Design review of the part shown in the three views and the two pictorial views. Dimensions are in mm from the part's minimum x, y and z. A direction names the side the tool comes from. Round coordinates to 2 decimals unless told otherwise and drop trailing zeros. Write each loop counter-clockwise with the first axis right and the second up, starting at its lowest first coordinate (ties: lowest second). Pieces come first, ordered by that corner, then holes. Notation, with made-up numbers: (10.5, -4) -> (24.5, -4) arc R26 cw to (24.5, 13) -> close; hole circle Ø5 at (-39.75, 50). An arc over 180 degrees is marked (long way). Return JSON: item names as keys, results as strings. Group by question number.
1. Take a section at A-A, the plane y = 6. Give the number of separate pieces and of enclosed holes in the cut face, then the cut area to 3 significant figures.
2. Tool access review of the marked faces 1 and 2: name each direction out of +Z, -Z, +X, -X, +Y, -Y from which nothing blocks a thin tool from reaching the whole face with its end or side.
3. Take a section at C-C, the plane z = 8.75. Write out the cut boundary in (x, y), then the cut area to 3 significant figures.
4. Clearance check with flat-ended pins moving along their axes: P1, Ø3.5, axis at x = 19.5, z = 7, coming from the -Y side; P2, Ø2.5, axis at x = 7, z = 5.5, coming from the +Y side; P3, Ø1, axis at y = 2, z = 1.5, coming from the -X side. State where each tip first meets the part, or that it passes through.
5. Mouldability with a two-part tool opening along X and no side actions: class the marked faces 3, 4 and 5 as pulls with the +X half, pulls with the -X half, needs draft (parallel to the pull), parting line crosses it, or undercut.
6. For line 1 along X through (y, z) = (13, 7); line 2 along Z through (x, y) = (19.5, 12.3); line 3 along X through (y, z) = (3.75, 6.25) (1 decimal), list the stretches that pass through material, from the lowest coordinate up. Write a range as from..to.
7. Take a section at B-B, the plane x = 13. Write out the cut boundary in (y, z).
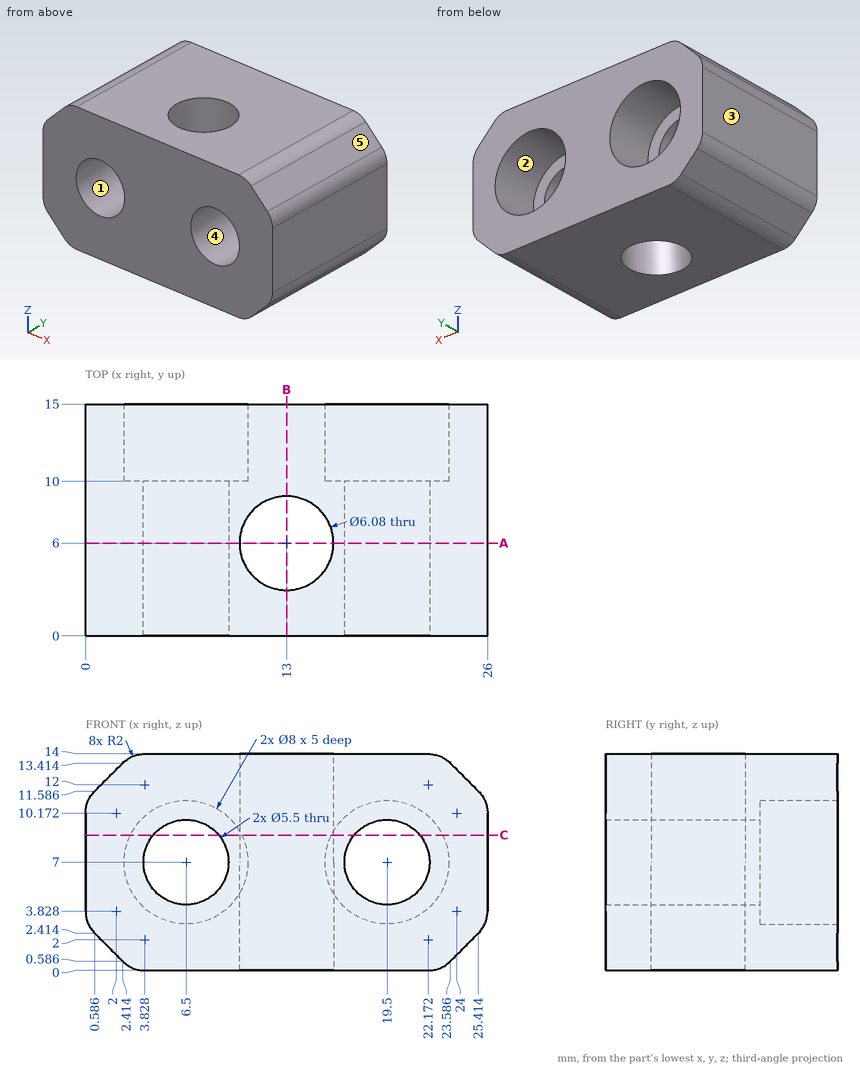
Output:
{
 "1": {"separate pieces": "2", "enclosed holes": "2", "area": "213 mm^2"},
 "2": {"face 1": "+Y, -Y", "face 2": "+Y"},
 "3": {"outline": "(0, 0) -> (4.38, 0) -> (4.38, 10) -> (2.9, 10) -> (2.9, 15) -> (0, 15) -> close; (8.62, 0) -> (17.38, 0) -> (17.38, 10) -> (15.9, 10) -> (15.9, 15) -> (10.1, 15) -> (10.1, 10) -> (8.62, 10) -> close; (21.62, 0) -> (26, 0) -> (26, 15) -> (23.1, 15) -> (23.1, 10) -> (21.62, 10) -> close; hole circle Ø6.08 at (13, 6)", "area": "204 mm^2"},
 "4": {"P1": "passes through", "P2": "stops at y = 10", "P3": "stops at x = 1"},
 "5": {"face 3": "pulls with the -X half", "face 4": "undercut", "face 5": "pulls with the +X half"},
 "6": {"line 1": "x = 0..2.5, 10.5..15.5, 23.5..26", "line 2": "z = 0..3, 11..14", "line 3": "x = 0..3.9, 9.1..11, 15..16.9, 22.1..26"},
 "7": {"outline": "(0, 0) -> (2.96, 0) -> (2.96, 14) -> (0, 14) -> close; (9.04, 0) -> (15, 0) -> (15, 14) -> (9.04, 14) -> close"}
}
